The drawing under review shows one solid part. Ordinate dimensions are in mm from its lowest x, y, z. A direction names the side the tool comes from. Give positions to 0.01 mm unless a question says otherwise; leave off trailing zeros. Write each loop counter-clockwise with the first axis right and the second up, starting at its lowest first coordinate (ties: lowest second). Pieces come first, ordered by that corner, then holes. Notation, with made-up numbers: (-17, -31.75) -> (15, -31.75) arc R27 cw to (15, -13.75) -> close; hole circle Ø4 at (11.25, 37). An arc over 180 degrees is marked (long way). Write item = value, one per line.
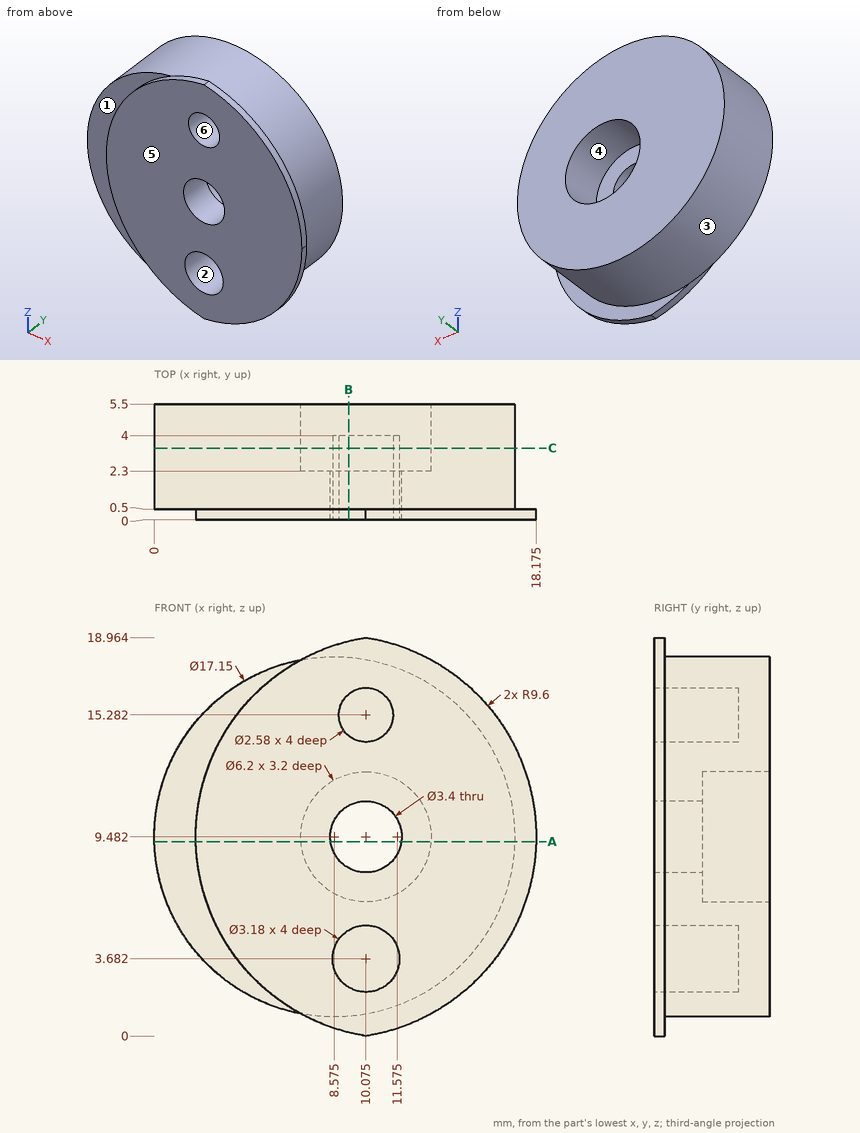
(1) Take a section at B-B (x = 9.25). Write out the cut boundary in (y, z).
Answers below:
outline = (0, 0.17) -> (0.5, 0.17) -> (0.5, 0.93) -> (5.5, 0.93) -> (5.5, 6.49) -> (2.3, 6.49) -> (2.3, 8) -> (0, 8) -> (0, 5.04) -> (4, 5.04) -> (4, 2.32) -> (0, 2.32) -> close; (0, 10.97) -> (2.3, 10.97) -> (2.3, 12.47) -> (5.5, 12.47) -> (5.5, 18.03) -> (0.5, 18.03) -> (0.5, 18.8) -> (0, 18.8) -> (0, 16.27) -> (4, 16.27) -> (4, 14.29) -> (0, 14.29) -> close
(2) The part is to be moulded in two halves that separate along X. For the marked faces 1, 2 and 3, say which applies: released by +X, released by -X, zero draft, split by the parting line, or undercut.
Answers below:
face_1 = zero draft
face_2 = undercut
face_3 = split by the parting line
(3) To check wall thickness, follow probe 1 along Z at (x, y) = (8.75, 2) (1 decimal); probe 2 along X at (y, z) = (2.15, 9.5) (3 decimals); probe 3 along Y at (x, z) = (7.5, 9.5). State the ranges of each line that lie inside material, in increasing order.
Answers below:
probe_1 = 0.9 to 2.8, 4.6 to 8.4, 10.5 to 18.1
probe_2 = 0 to 8.375, 11.775 to 17.15
probe_3 = 0 to 2.3
(4) Take a section at C-C (y = 3.4). Count the separate pieces of the cut face and the enclosed holes in it, plus the area to 3 significant figures.
Answers below:
separate_pieces = 1
enclosed_holes = 3
area = 188 mm^2
(5) For pin 1 (7 mm diameter, centred on x = 10.07, z = 9.48, fed in from -Y); pin 2 (2.5 mm diameter, centred on x = 10.07, z = 9.48, fed in from +Y); pin 3 (1 mm diameter, centred on x = 13.5, y = 2.5, fed in from -Z); pin 4 (2.5 mm diameter, centred on x = 10, z = 3.5, fed in from -Y), all flat-tipped, find the tip position at first contact; note any pin that passes through.
Answers below:
pin_1 = 0
pin_2 = through
pin_3 = 2.14
pin_4 = 4
(6) Tool access review of the marked faces 4, 5 and 6: name each direction out of +Z, -Z, +X, -X, +Y, -Y from which nothing blocks a thin tool from reaching the whole face with its end or side.
Answers below:
face_4 = +Y
face_5 = +Z, -Z, +X, -X, -Y
face_6 = -Y
(7) Take a section at A-A (z = 9.25). Write out the cut boundary in (x, y), plus the area to 3 significant figures.
Answers below:
outline = (0, 0.5) -> (1.98, 0.5) -> (1.98, 0) -> (8.39, 0) -> (8.39, 2.3) -> (6.98, 2.3) -> (6.98, 5.5) -> (0, 5.5) -> close; (11.76, 0) -> (18.17, 0) -> (18.17, 0.5) -> (17.15, 0.5) -> (17.15, 5.5) -> (13.17, 5.5) -> (13.17, 2.3) -> (11.76, 2.3) -> close
area = 66.3 mm^2
